Input: part model. Units: mm. Frame: model coordinates. Coordinates: 2 decimals unless noted, no trailing zeros. Loops run counter-clockwise (first coordinate to the right, second up) from the corner with the lowest first, then second, coordinate; pieces in that order, holes last.
```python
from build123d import *

# Parameters (mm, degrees)
F0_W          = 22.352
F0_H          = 1.27
F1_DEPTH      = 38.1
F2_W          = 6.8990886211
F2_H          = 17.6976025105
F3_DEPTH      = 25.4
F3_DEPTH_BACK = 25.4


with BuildPart() as f1:
    # F0 (on Right) → F1 (new body)
    with BuildSketch(Plane.YZ):
        Rectangle(F0_W, F0_H)
    extrude(amount=F1_DEPTH)

    # F2 (on Top) → F3 (cut, two sides)
    with BuildSketch(Plane.XY) as f3_sk:
        with Locations((26.0965079069, 0)):
            Rectangle(F2_W, F2_H)
    extrude(amount=-F3_DEPTH, mode=Mode.SUBTRACT)
    extrude(f3_sk.sketch, amount=F3_DEPTH_BACK, mode=Mode.SUBTRACT)


solid = f1.part
```
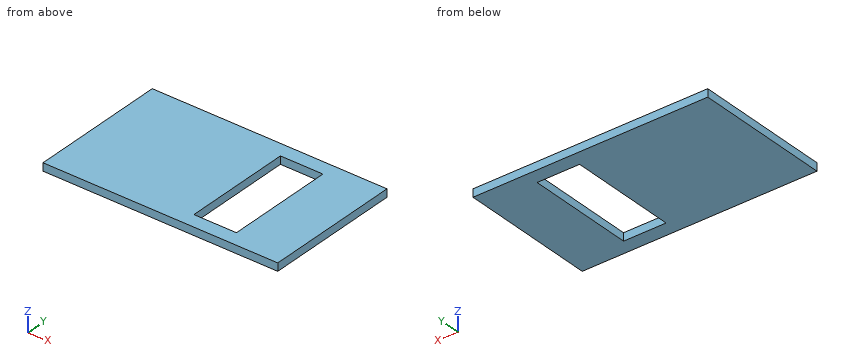
Item 1: Section query A-A (z = 0.35). Output: boundary loops of the cut face in (x, y).
Result:
outline: (0, -11.18) - (38.1, -11.18) - (38.1, 11.18) - (0, 11.18) - close; hole (22.65, -8.85) - (29.55, -8.85) - (29.55, 8.85) - (22.65, 8.85) - close
Item 2: Line query: L1, parallel to Y at x = 24, z = 0.25; L2, parallel to X at y = -4.5, z = 0.2. Output: solid intervals per line, ascending.
Result:
L1: y = -11.18 to -8.85, 8.85 to 11.18
L2: x = 0 to 22.65, 29.55 to 38.1
Item 3: Section query C-C (x = 27). Output: boundary loops of the cut face in (y, z) (3 decimals).
Result:
outline: (-11.176, -0.635) - (-8.849, -0.635) - (-8.849, 0.635) - (-11.176, 0.635) - close; (8.849, -0.635) - (11.176, -0.635) - (11.176, 0.635) - (8.849, 0.635) - close
Item 4: Section query B-B (y = 8). Output: boundary loops of the cut face in (x, z) (3 decimals).
Result:
outline: (0, -0.635) - (22.647, -0.635) - (22.647, 0.635) - (0, 0.635) - close; (29.546, -0.635) - (38.1, -0.635) - (38.1, 0.635) - (29.546, 0.635) - close
